Source: three-view drawing plus pictorial views. Frame: mm from the lowest corner of the part. A direction names the side the tool comes from. Give positions to 0.01 mm unless a question says otherwise; leave off trailing zeros. Loops run counter-clockwise (first coordinate to the right, second up) from the corner with the lowest first, then second, coordinate; pieces in that order, holes last. Notation, with made-up numbers: M 26,-23.75 L 80,-23.75 A21 ccw 80,-15.75 Z; hole C -31.75,45.5 d5. An arc over 180 degrees is marked long. Write item = value, one per line.
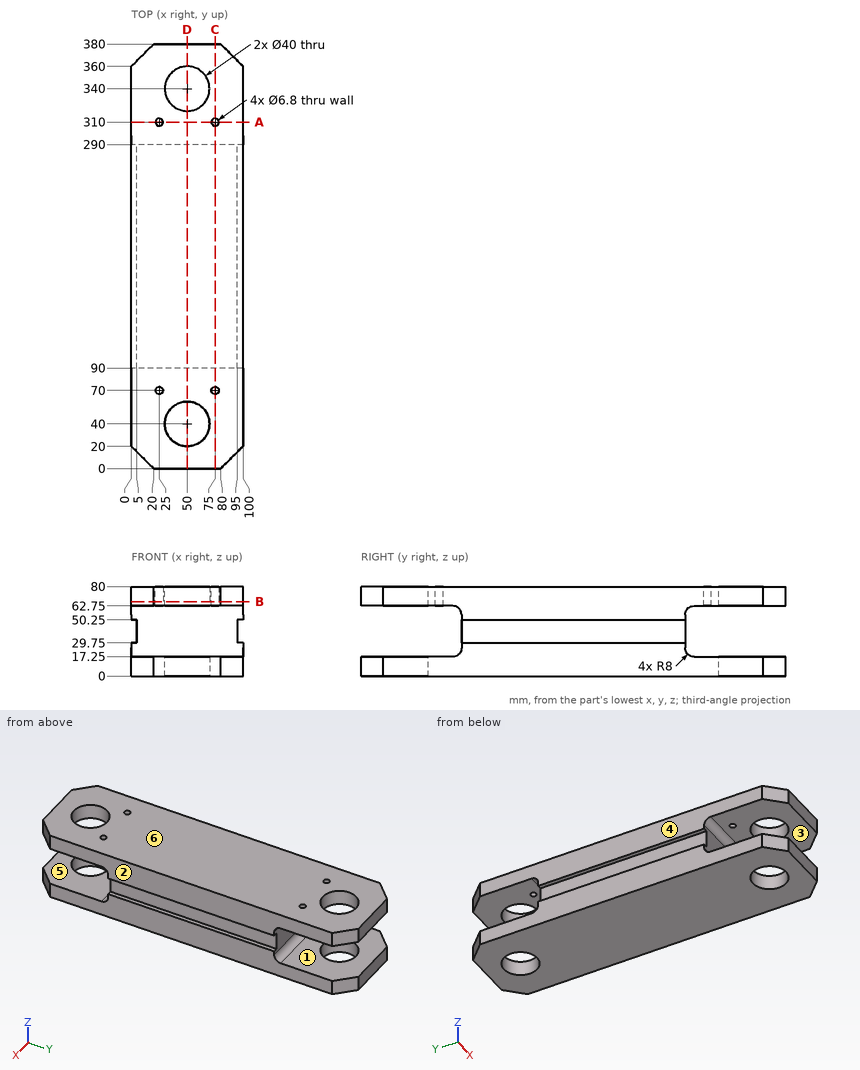
1. Material intervals for probe 1 along X at (y, z) = (310, 72.75); probe 2 along Y at (x, z) = (25, 67.75); probe 3 along Y at (x, z) = (50, 10.5), sorted ascending. Write a range as from..to.
Derived:
probe_1 = 0..21.6, 28.4..71.6, 78.4..100
probe_2 = 0..66.6, 73.4..306.6, 313.4..380
probe_3 = 0..20, 60..320, 360..380
2. Cut plane A-A, the plane y = 310. Return the cut outline in (x, z), then the cut area to 3 significant figures.
Derived:
outline = M 0,0 L 100,0 L 100,17.25 L 0,17.25 Z; M 0,62.75 L 21.6,62.75 L 21.6,80 L 0,80 Z; M 28.4,62.75 L 71.6,62.75 L 71.6,80 L 28.4,80 Z; M 78.4,62.75 L 100,62.75 L 100,80 L 78.4,80 Z
area = 3,220 mm²
3. Cut plane D-D, the plane x = 50. Count the separate pieces of the cut face and the enclosed holes in it, then the cut area to 3 significant figures.
Derived:
separate_pieces = 5
enclosed_holes = 0
area = 19,500 mm²
4. First-contact query: pin 1 Ø16.5 at (y, z) = (186, 39.5) entering from +X; pin 2 Ø4 at (x, y) = (75, 70) entering from +Z; pin 3 Ø23.5 at (x, z) = (39.5, 47) entering from -Y. Flat tips, straight axial feed; report the tip coordinate or a pass-through.
Derived:
pin_1 = 95
pin_2 = 17.25
pin_3 = 88.93
5. Cut plane B-B, the plane z = 66.5. Return the cut outline in (x, y).
Derived:
outline = M 0,20 L 20,0 L 80,0 L 100,20 L 100,360 L 80,380 L 20,380 L 0,360 Z; hole C 25,70 d6.8; hole C 25,310 d6.8; hole C 50,40 d40; hole C 50,340 d40; hole C 75,70 d6.8; hole C 75,310 d6.8
6. Cut plane C-C, the plane x = 75. Return the cut outline in (y, z).
Derived:
outline = M 0,0 L 380,0 L 380,17.25 L 298,17.25 A8 cw 290,25.25 L 290,54.75 A8 cw 298,62.75 L 306.6,62.75 L 306.6,80 L 73.4,80 L 73.4,62.75 L 82,62.75 A8 cw 90,54.75 L 90,25.25 A8 cw 82,17.25 L 0,17.25 Z; M 0,62.75 L 66.6,62.75 L 66.6,80 L 0,80 Z; M 313.4,62.75 L 380,62.75 L 380,80 L 313.4,80 Z
7. Pull-direction query (Z, two-part tool) for the marked faces 3, 4, 5 and 6; classes: +Z half, -Z half, draft (parallel to the pull), parting line (faces both ways), or undercut.
Derived:
face_3 = undercut
face_4 = draft
face_5 = undercut
face_6 = +Z half
8. Reachability of the marked faces 1 and 2 from +Z, -Z, +X, -X, +Y, -Y: full face, straight path, thin tool, end or side. Return the list, or none.
Derived:
face_1 = +X, -X, +Y
face_2 = +Z, -Z, +X, +Y, -Y
